Model file for the job. Use its own axes, mm. A direction names the side the tool comes from. Round coordinates to 2 decimals unless told otherwise and drop trailing zeros. Loops run counter-clockwise (first coordinate to the right, second up) from the corner with the lowest first, then second, coordinate; pieces in that order, holes last. Notation, with made-up numbers: M 5.25,11.25 L 21.25,11.25 A30 cw 21.25,48.25 Z; hole C -36.75,22.25 d10. An arc over 180 degrees is marked long. Use a Markdown table: item, result. Add a question column.
Item 1: Saw through at D-D on z = 107.5. Write the cut outline in (x, y).
Item 2: Wall check: L1, parallel to Z at x = 0, y = -38.25; L2, parallel to Y at x = -43, z = 67; L3, parallel to Z at x = -27, y = 30. Give the ranges that are in metal, low to high. Write a range as from..to.
Item 3: Pin check, flat tips, straight feed: P1, Ø3, axis at y = 1.5, z = -3, coming from the -X side; P2, Ø4, axis at x = -18, y = 37.5, coming from the -Z side; P3, Ø6, axis at y = -24.5, z = 13.5, coming from the +X side. Stop position of each tip, or through.
Item 4: Saw through at B-B on z = 92. Write the cut outline in (x, y).
Item 5: Saw through at A-A on z = 37.5. Write the cut outline in (x, y).
Item 6: Saw through at C-C on z = -9. Write the cut outline in (x, y).
Item 7: Tool access for faces 1 (the flat face through (38, 40, 20)), 2 (the flat face through (-1, -35, 58)), 3 (the flat face through (-40, -38, 20)), 4 (the flat face through (40, -40, 20)), 5 (the cylindrical face through (47.69, 15.02, 10.87)): list every direction of +Z, -Z, +X, -X, +Y, -Y with a clear straight run to the whole face (end or side of a thin tool).
Item 8: Two-plate mould, pull along Y, no slides. Class faces 6 (the flat face through (-1, 0, 30)), 7 (the flat face through (-11.8, 50, 63.5)), 8 (the flat face through (21, 1, 0)): +Y half, -Y half, draft (parallel to the pull), parting line (faces both ways), or undercut.
```python
from build123d import *

# Parameters (mm, degrees)
SKETCH_R        = 50
PAD_DEPTH       = 20
CHAMFER_SIZE    = 2
SKETCH001_R     = 18
PAD001_DEPTH    = 20
SKETCH002_W     = 100
SKETCH002_H     = 100
PAD002_DEPTH    = 10
PAD003_DEPTH    = 50
SKETCH004_R     = 20
POCKET_DEPTH    = 101
SKETCH005_W     = 100
SKETCH005_H     = 101
POCKET001_DEPTH = 35


with BuildPart() as part:
    # Sketch → Pad (new body)
    with BuildSketch(Plane.XY):
        Circle(SKETCH_R)
    extrude(amount=PAD_DEPTH)

    # Chamfer
    chamfer_edges = [part.edges().sort_by_distance(p)[0] for p in [
        (-50, 0, 0),
    ]]
    chamfer(chamfer_edges, length=CHAMFER_SIZE)

    # Sketch001 (on Face4 of Chamfer) → Pad001 (join)
    with BuildSketch(Plane(origin=(0, 0, 0), x_dir=(1, 0, 0), z_dir=(0, 0, -1))):
        Circle(SKETCH001_R)
    extrude(amount=PAD001_DEPTH)

    # Sketch002 (on Face3 of Pad001) → Pad002 (join)
    with BuildSketch(Plane.XY.offset(20)):
        Rectangle(SKETCH002_W, SKETCH002_H)
    extrude(amount=PAD002_DEPTH)

    # Sketch003 → Pad003 (join, symmetric)
    with BuildSketch(Plane.XZ):
        with BuildLine():
            ThreePointArc((50, 80), (0, 130), (-50, 80))
            Line((-50, 30), (-50, 80))
            Line((50, 30), (-50, 30))
            Line((50, 80), (50, 30))
        make_face()
    extrude(amount=PAD003_DEPTH, both=True)

    # Sketch004 (on Face13 of Pad003) → Pocket (cut)
    with BuildSketch(Plane.XZ.offset(50)):
        with Locations((0, 80)):
            Circle(SKETCH004_R)
    extrude(amount=-POCKET_DEPTH, mode=Mode.SUBTRACT)

    # Sketch005 → Pocket001 (cut, symmetric)
    with BuildSketch(Plane.XZ):
        with Locations((0, 80.5)):
            Rectangle(SKETCH005_W, SKETCH005_H)
    extrude(amount=POCKET001_DEPTH, both=True, mode=Mode.SUBTRACT)


solid = part.part
```
Entries:
| question | item | result |
|---|---|---|
| 1 | outline | M -41.76,-50 L 41.76,-50 L 41.76,-35 L -41.76,-35 Z; M -41.76,35 L 41.76,35 L 41.76,50 L -41.76,50 Z |
| 2 | L1 | 0..60, 100..130 |
| 2 | L2 | -50..-35, 35..50 |
| 2 | L3 | 0..30 |
| 3 | P1 | x = -18 |
| 3 | P2 | z = 0 |
| 3 | P3 | x = 45.14 |
| 4 | outline | M -48.54,-50 L -16,-50 L -16,-35 L -48.54,-35 Z; M -48.54,35 L -16,35 L -16,50 L -48.54,50 Z; M 16,-50 L 48.54,-50 L 48.54,-35 L 16,-35 Z; M 16,35 L 48.54,35 L 48.54,50 L 16,50 Z |
| 5 | outline | M -50,-50 L 50,-50 L 50,-35 L -50,-35 Z; M -50,35 L 50,35 L 50,50 L -50,50 Z |
| 6 | outline | C 0,0 d36 |
| 7 | face 1 | -Z, +X, +Y |
| 7 | face 2 | +Z, +X, -X |
| 7 | face 3 | -Z, -X, -Y |
| 7 | face 4 | -Z, +X, -Y |
| 7 | face 5 | -Z |
| 8 | face 6 | undercut |
| 8 | face 7 | +Y half |
| 8 | face 8 | draft |
